```python
from build123d import *

# Parameters (mm, degrees)
SKETCH1_W           = 50
SKETCH1_H           = 100
BOSS_EXTRUDE1_DEPTH = 7
CUT_EXTRUDE1_DEPTH  = 10
CUT_EXTRUDE2_DEPTH  = 28
SKETCH5_W           = 3
SKETCH5_H           = 4.633494333
SKETCH5_H_2         = 4.765216978
BOSS_EXTRUDE2_DEPTH = 15
SKETCH6_R           = 2.1
CUT_EXTRUDE3_DEPTH  = 15
CHAMFER1_SIZE       = 3
CUT_EXTRUDE4_DEPTH  = 3
FILLET1_R           = 5
SKETCH8_W           = 66.498468349
SKETCH8_H           = 65.695900627
CUT_EXTRUDE5_DEPTH  = 29


with BuildPart() as part:
    # Sketch1 → Boss-Extrude1 (new body)
    with BuildSketch(Plane(origin=(0, 0, 0), x_dir=(1, 0, 0), z_dir=(0, 1, 0))):
        with Locations((-16.984615004, 32.878894954)):
            Rectangle(SKETCH1_W, SKETCH1_H)
    extrude(amount=BOSS_EXTRUDE1_DEPTH)

    # Sketch2 → Cut-Extrude1 (cut)
    with BuildSketch(Plane.XZ):
        Polygon((8.015384996, -49.878894954), (6.015384996, -49.878894954), (-18.491384598, -49.878894954), (-18.491384598, -50.378894954), (-18.491384598, -65.378894954), (-28.491384598, -65.378894954), (-28.491384598, -50.378894954), (-28.491384598, -49.878894954), (-39.984615004, -49.878894954), (-41.984615004, -49.878894954), (-41.984615004, -82.878894954), (8.015384996, -82.878894954), align=None)
    extrude(amount=-CUT_EXTRUDE1_DEPTH, mode=Mode.SUBTRACT)

    # Sketch4 → Cut-Extrude2 (cut)
    with BuildSketch(Plane.XZ):
        Polygon((8.015384996, -42.228894954), (-0.484615004, -42.228894954), (-33.484615004, -42.228894954), (-41.984615004, -42.228894954), (-41.984615004, -45.228894954), (-33.484615004, -45.228894954), (-0.484615004, -45.228894954), (8.015384996, -45.228894954), align=None)
    extrude(amount=-CUT_EXTRUDE2_DEPTH, mode=Mode.SUBTRACT)


with BuildPart() as cut_extrude2_piece_1:
    # of the separate pieces the step leaves, piece 1, a body of its own (cut_extrude2_pieces)
    add(part.part.solids().sort_by_distance((8.015384996, 0, 17.121105046))[0])

    # Sketch8 → Cut-Extrude5 (cut)
    with BuildSketch(Plane(origin=(0, 7, 0), x_dir=(1, 0, 0), z_dir=(0, 1, 0))):
        with Locations((-10.449420701, 11.294291779)):
            Rectangle(SKETCH8_W, SKETCH8_H)
    extrude(amount=-CUT_EXTRUDE5_DEPTH, mode=Mode.SUBTRACT)


with BuildPart() as cut_extrude2_piece_2:
    # of the separate pieces the step leaves, piece 2, a body of its own (cut_extrude2_pieces)
    add(part.part.solids().sort_by_distance((8.015384996, 0, -49.878894954))[0])

    # Sketch5 → Boss-Extrude2 (add)
    with BuildSketch(Plane(origin=(0, 7, 0), x_dir=(1, 0, 0), z_dir=(0, 1, 0))):
        with Locations((9.515384996, 47.545642121)):
            Rectangle(SKETCH5_W, SKETCH5_H)
        with Locations((-43.484615004, 47.611503443)):
            Rectangle(SKETCH5_W, SKETCH5_H_2)
    extrude(amount=-BOSS_EXTRUDE2_DEPTH)

    # Sketch6 → Cut-Extrude3 (cut)
    with BuildSketch(Plane(origin=(0, 7, 0), x_dir=(1, 0, 0), z_dir=(0, 1, 0))):
        with Locations(Location((-23.491299754, 57.878894954, 0), (0, 0, 270))):
            Circle(SKETCH6_R)
    extrude(amount=-CUT_EXTRUDE3_DEPTH, mode=Mode.SUBTRACT)

    # Chamfer1
    chamfer1_edges = [cut_extrude2_piece_2.edges().sort_by_distance(p)[0] for p in [
        (-28.491384598, 3.5, -65.378894954),
        (-18.491384598, 3.5, -65.378894954),
    ]]
    chamfer(chamfer1_edges, length=CHAMFER1_SIZE)

    # Sketch7 → Cut-Extrude4 (cut)
    with BuildSketch(Plane(origin=(0, 7, 0), x_dir=(1, 0, 0), z_dir=(0, 1, 0))):
        with BuildLine():
            Line((-28.491384598, 55.878894954), (-27.522428628, 55.878894954))
            ThreePointArc((-27.522428628, 55.878894954), (-23.491299754, 53.378894954), (-19.46017088, 55.878894954))
            Line((-19.46017088, 55.878894954), (-18.491384598, 55.878894954))
            Line((-18.491384598, 55.878894954), (-18.491384598, 59.878894954))
            Line((-18.491384598, 59.878894954), (-19.46017088, 59.878894954))
            ThreePointArc((-19.46017088, 59.878894954), (-23.491299754, 62.378894954), (-27.522428628, 59.878894954))
            Line((-27.522428628, 59.878894954), (-28.491384598, 59.878894954))
            Line((-28.491384598, 59.878894954), (-28.491384598, 55.878894954))
        make_face()
    extrude(amount=-CUT_EXTRUDE4_DEPTH, mode=Mode.SUBTRACT)

    # Fillet1
    # the kernel refuses this fillet: 5 mm, written as the material it takes off along each edge
    with BuildSketch(Plane(origin=(-21.491384598, -5.17766953, -65.378894954), x_dir=(0.7071067811865483, 0, 0.7071067811865466), z_dir=(0, 1, 0)), Plane(origin=(-25.491384598, -5.17766953, -65.378894954), x_dir=(1, 0, 0), z_dir=(0, 1, 0))) as fillet1_piece_1:
        with BuildLine():
            CenterArc((FILLET1_R * 0.414213562373, -FILLET1_R), FILLET1_R, 90, 45)
            Line((-FILLET1_R * 0.292893218813, -FILLET1_R * 0.292893218813), (0, 0))
            Line((0, 0), (FILLET1_R * 0.414213562373, 0))
        make_face()
    extrude(amount=17.355339059, mode=Mode.SUBTRACT)


solid = cut_extrude2_piece_2.part
```
The listing builds one solid part. Answer for the finished solid, in the listing's coordinates (mm). A direction names the side the tool comes from. Coordinates: 2 decimals unless noted, no trailing zeros. Loops run counter-clockwise (first coordinate to the right, second up) from the corner with the lowest first, then second, coordinate; pieces in that order, holes last. Notation, with made-up numbers: M 53,77 L 74,77 A10 cw 74,93 Z; hole C 23,59.25 d2. An arc over 180 degrees is marked long. Answer as CSV lines item,"result". Start each with the question number.
(1) Find the intervals of material crossed by L1, parallel to X at y = 3, z = -57.75; L2, parallel to Y at x = -12, z = -49.75; L3, parallel to Z at x = -8.5, y = 6, in increasing order. Write a range as [from, to].
(2) The part is cut by section C-C (z = -47.25). Give the vertices of the cut face in (x, y).
(3) The part is cut by section D-D (x = -22). Give the vertices of the cut face in (y, z), and give its area (3 significant figures).
(4) The mould has two halves that part along Z. Classify faces 6 (the flat face through (11.015, 0, -48)), 7 (the cylindrical face through (-23.56, 5.52, -53.38)), 8 (the flat face through (-5, 3, -49.879)), 9 (the flat face through (-22, 4, -56)): pulls with the +Z half, pulls with the -Z half, needs draft (parallel to the pull), parting line crosses it, or undercut.
(5) Given pin 1 (0.9 mm diameter, centred on x = -43, y = 3, fed in from -Z); pin 2 (4.5 mm diameter, centred on x = -24.5, z = -59.5, fed in from +Y); pin 3 (7.5 mm diameter, centred on y = 4.5, z = -57.5, fed in from -X); pin 4 (8 mm diameter, centred on y = -5, z = -54.5, fed in from -X), each flat-ended and moving along its own axis, determine where each tip first touches the part or whether it passes through.
(6) For faces 1 (the cylindrical face through (-23.42, 5.52, -62.38)), 2 (the flat face through (-28, 6, -55.879)), 3 (the flat face through (-23, 0, -51)), 4 (the flat face through (-35, 3, -49.879)), 5 (the flat face through (9, 0, -49.862)), determine the directions among +Z, -Z, +X, -X, +Y, -Y from which every point of the face is accessible in a straight line to the end or side of a thin tool.
(7) The part is cut by section B-B (z = -56.5). Give the vertices of the cut face in (x, y).
Determined:
1,L1,"[-28.49, -25.59], [-21.4, -18.49]"
1,L2,"[0, 7]"
1,L3,"[-49.88, -45.23]"
2,outline,"M -44.98,-8 L -41.98,-8 L -41.98,0 L 8.02,0 L 8.02,-8 L 11.02,-8 L 11.02,7 L -44.98,7 Z"
3,outline,"M 0,-65.13 L 7,-65.13 L 7,-62.12 L 4,-62.12 L 4,-59.36 L 0,-59.36 Z; M 0,-56.4 L 4,-56.4 L 4,-53.63 L 7,-53.63 L 7,-45.23 L 0,-45.23 Z"
3,area,"102 mm2"
4,face 6,"needs draft"
4,face 7,"undercut"
4,face 8,"pulls with the -Z half"
4,face 9,"undercut"
5,pin 1,"z = -49.99"
5,pin 2,"y = 4"
5,pin 3,"x = -28.49"
5,pin 4,"through"
6,face 1,"+Y"
6,face 2,"+X, -X, +Y"
6,face 3,"+Z, -Z, -Y"
6,face 4,"-Z, +Y, -Y"
6,face 5,"-Z, +X, +Y, -Y"
7,outline,"M -28.49,0 L -25.08,0 L -25.08,4 L -28.49,4 Z; M -21.91,0 L -18.49,0 L -18.49,4 L -21.91,4 Z"
